Can you work these out from the model? Positions are in its coordinate system, mm. A direction names the side the tool comes from. Give positions to 0.01 mm unless a question says otherwise; leave off trailing zeros. Order: outer loops, then holes, each group sorted by start corner. A loop starts at its lowest first (then second) coordinate and runs counter-clockwise, first axis right, second up. Notation, with made-up numbers: M 4.5,-11 L 46.5,-11 A28 cw 46.5,16 Z; hole C 28,15 d6. An arc over 180 degrees is marked long. Use a Markdown table: item, result. Add a question column.
from build123d import *

# Parameters (mm, degrees)
F0_W     = 10
F0_H     = 20
F1_DEPTH = 10
F2_W     = 2.2
F2_H     = 6
F3_DEPTH = 8.2
F4_R     = 2.05
F5_DEPTH = 3
F6_D     = 3.6
F8_D     = 3.6


with BuildPart() as f1:
    # F0 (on Front) → F1 (new body)
    with BuildSketch(Plane.XZ):
        with Locations((-0.0625, 0)):
            Rectangle(F0_W, F0_H)
    extrude(amount=F1_DEPTH)

    # F2 (on face) → F3 (cut)
    with BuildSketch(Plane(origin=(0, 0, 0), x_dir=(-1, 0, 0), z_dir=(0, 1, 0))):
        with Locations((0, 6.15)):
            Rectangle(F2_W, F2_H)
        with Locations((0, -6.15)):
            Rectangle(F2_W, F2_H)
    extrude(amount=-F3_DEPTH, mode=Mode.SUBTRACT)

    # F4 (on face) → F5 (cut)
    with BuildSketch(Plane.XZ.offset(10)):
        Circle(F4_R)
    extrude(amount=-F5_DEPTH, mode=Mode.SUBTRACT)

    # F6 (through all)
    with Locations(Plane(origin=(0, 0, 0), x_dir=(1, 0, 0), z_dir=(0, 1, 0))):
        with Locations((0, 0)):
            Hole(F6_D / 2)

    # F8 (through all)
    with Locations(Plane.YZ.offset(4.9375)):
        with Locations((-5, -6.15), (-5, 6.15)):
            Hole(F8_D / 2)


solid = f1.part
1. If we section it at B-B, the plane y = -5: State how many separate pieces and enclosed holes the cut face has, then the cut area to 3 significant figures.
2. Will these pins go through, and if not, where does the flat tip stop? pin 1 (3 mm diameter, centred on y = -5, z = 6.15, fed in from +X); pin 2 (1.8 mm diameter, centred on x = 0.5, z = -7, fed in from +Y).
3. I need wall thicknesses on L1, parallel to Z at x = -3.4, y = -5; L2, parallel to Z at x = -0.75, y = -1.5; L3, parallel to X at y = -0.75, z = 7.5. Which ranges of each line are inside material? Lowest first, please. Write a range as [from, to].
4. On a 3-axis mill with a long thin cutter (end or side, diameter ignored), from which of +Z, -Z, +X, -X, +Y, -Y can I reach the whole of each face in a straight line? I mean faces 1 (the face through (-2, 0, 0)), 2 (the face through (1.1, -3, 6)). Say none if no direction works.
5. If we section it at A-A, the plane x = 0: List the corners of the cut face in (y, z) for me, then the cut area to 3 significant figures.
6. If we section it at C-C, the plane z = 0: List the corners of the cut face in (x, y) for me, then the cut area to 3 significant figures.
7. We'd pull the mould along Y, two halves only. Please class faces 3 (the face through (-1.717, -3.549, -0.541)), 4 (the face through (-0.1, -10, 2.4)), 5 (the face through (2.992, -5.968, 7.668)): +Y half, -Y half, draft (parallel to the pull), parting line (faces both ways), or undercut.
8. If we section it at D-D, the plane x = -1.5: List the corners of the cut face in (y, z) for me.
Geometry results:
| question | item | result |
|---|---|---|
| 1 | separate pieces | 3 |
| 1 | enclosed holes | 1 |
| 1 | area | 107 mm^2 |
| 2 | pin 1 | passes through |
| 2 | pin 2 | stops at y = 0 |
| 3 | L1 | z = [-10, -7.95], [-4.35, 4.35], [7.95, 10] |
| 3 | L2 | z = [-10, -9.15], [-3.15, -1.64], [1.64, 3.15], [9.15, 10] |
| 3 | L3 | x = [-5.06, -1.1], [1.1, 4.94] |
| 4 | face 1 | +Z, -Z, +X, -X, +Y |
| 4 | face 2 | +Y |
| 5 | outline | M -10,-10 L 0,-10 L 0,-9.15 L -8.2,-9.15 L -8.2,-3.15 L 0,-3.15 L 0,-1.8 L -7,-1.8 L -7,-2.05 L -10,-2.05 Z; M -10,2.05 L -7,2.05 L -7,1.8 L 0,1.8 L 0,3.15 L -8.2,3.15 L -8.2,9.15 L 0,9.15 L 0,10 L -10,10 Z |
| 5 | area | 64.1 mm^2 |
| 6 | outline | M -5.06,-10 L -2.05,-10 L -2.05,-7 L -1.8,-7 L -1.8,0 L -5.06,0 Z; M 1.8,-7 L 2.05,-7 L 2.05,-10 L 4.94,-10 L 4.94,0 L 1.8,0 Z |
| 6 | area | 62.5 mm^2 |
| 7 | face 3 | draft |
| 7 | face 4 | -Y half |
| 7 | face 5 | undercut |
| 8 | outline | M -10,-10 L 0,-10 L 0,-0.99 L -7,-0.99 L -7,-1.4 L -10,-1.4 Z; M -10,1.4 L -7,1.4 L -7,0.99 L 0,0.99 L 0,10 L -10,10 Z; hole C -5,-6.15 d3.6; hole C -5,6.15 d3.6 |
